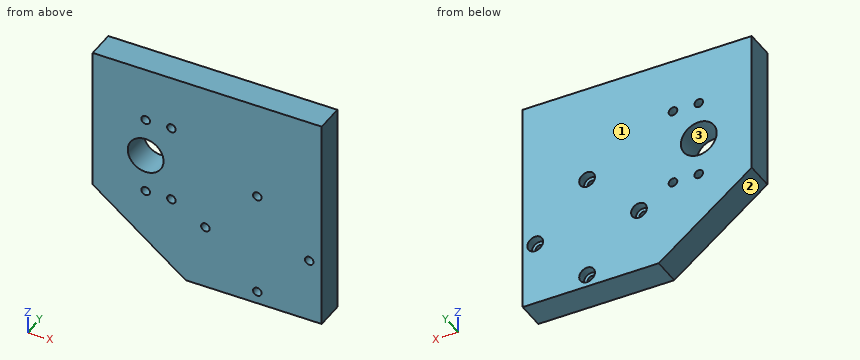
from build123d import *

# Parameters (mm, degrees)
F0_R     = 18
F0_R_2   = 3
F0_W     = 3
F0_H     = 17
F0_H_2   = 27
F0_R_3   = 12.5
F1_DEPTH = 20
F2_DEPTH = 25
F3_R     = 3
F4_DEPTH = 25
F5_R     = 5.5
F6_DEPTH = 6


with BuildPart() as f1:
    # F0 (on Front) → F1 (new body)
    with BuildSketch(Plane.XZ):
        Polygon((60, 50), (60, 0), (155, 0), (155, 90), (63, 90), (63, 63), (60, 63), align=None)
        Polygon((1, 63), (60, 63), (60, 90), (60, 107), (1, 107), align=None)
        with Locations((32, 85)):
            Circle(F0_R, mode=Mode.SUBTRACT)
        Polygon((-5, 50), (60, 50), (60, 63), (1, 63), (1, 107), (60, 107), (60, 120), (-5, 120), align=None)
        with Locations((32, 58)):
            Circle(F0_R_2, mode=Mode.SUBTRACT)
        with Locations((50, 58)):
            Circle(F0_R_2, mode=Mode.SUBTRACT)
        with Locations((32, 112)):
            Circle(F0_R_2, mode=Mode.SUBTRACT)
        with Locations((50, 112)):
            Circle(F0_R_2, mode=Mode.SUBTRACT)
        Polygon((63, 90), (155, 90), (155, 150), (-5, 150), (-5, 120), (60, 120), (60, 107), (63, 107), align=None)
        with Locations((61.5, 98.5)):
            Rectangle(F0_W, F0_H)
        with Locations((61.5, 76.5)):
            Rectangle(F0_W, F0_H_2)
        with Locations((32, 85)):
            Circle(F0_R_3)
        with Locations((32, 85)):
            Circle(F0_R)
        with Locations((32, 85)):
            Circle(F0_R_3, mode=Mode.SUBTRACT)
        Polygon((-5, 50), (60, 0), (60, 50), align=None)
    extrude(amount=F1_DEPTH)

    # F0 (on Front) → F2 (cut)
    with BuildSketch(Plane.XZ):
        with Locations((32, 85)):
            Circle(F0_R_3)
    extrude(amount=F2_DEPTH, mode=Mode.SUBTRACT)

    # F3 (on face) → F4 (cut)
    with BuildSketch(Plane.XZ.offset(20)):
        with Locations((110, 81.25)):
            Circle(F3_R)
        with Locations((146.25, 45)):
            Circle(F3_R)
        with Locations((73.75, 45)):
            Circle(F3_R)
        with Locations((110, 8.75)):
            Circle(F3_R)
    extrude(amount=-F4_DEPTH, mode=Mode.SUBTRACT)

    # F5 (on face) → F6 (cut)
    with BuildSketch(Plane(origin=(0, 0, 0), x_dir=(-1, 0, 0), z_dir=(0, 1, 0))):
        with Locations((-146.25, 45)):
            Circle(F5_R)
        with Locations((-110, 81.25)):
            Circle(F5_R)
        with Locations((-73.75, 45)):
            Circle(F5_R)
        with Locations((-110, 8.75)):
            Circle(F5_R)
    extrude(amount=-F6_DEPTH, mode=Mode.SUBTRACT)


solid = f1.part
Check sheet for the modelled part. Datum: model origin and axes. Units: mm. Face numbers are marked on the shaded views. Round coordinates to 2 decimals unless told otherwise and drop trailing zeros. Order: outer loops, then holes, each group sorted by start corner. A loop starts at its lowest first (then second) coordinate and runs counter-clockwise, first axis right, second up. Notation, with made-up numbers: M 34.5,60.25 L 72.5,60.25 A20 cw 72.5,76.25 Z; hole C 21,35.25 d10. An arc over 180 degrees is marked long. One line per item, written item: value. Start each with the question number.
1. Scan lines: line 1 along Z through (x, y) = (110, -15); line 2 along Z through (x, y) = (146.25, -15.25); line 3 along Z through (x, y) = (50, -8). Record each from-to range of solid material in increasing order.
2. Section check B-B on y = -10.5. Give the number of separate pieces and of enclosed holes in the cut face, and give its area (3 significant figures).
3. Gauge pin test, flat ends, axial feed: P1, Ø15, axis at x = 32, z = 85, coming from the +Y side; P2, Ø9, axis at x = 73.75, z = 45, coming from the +Y side. Record the tip position at first contact, or that the pin passes through.
4. Section check C-C on x = 73.75. Enter the section's corners in (y, z).
5. Section check A-A on z = 45. Enter the section's corners in (x, y), and give its area (3 significant figures).
6. Section check D-D on x = 110. Enter the section's corners in (y, z).
7. Release check for a two-part mould opening along X. For the marked faces 1, 2 and 3 record: released by +X, released by -X, zero draft, split by the parting line, or undercut.
Results found:
1. line 1: 0 to 5.75, 11.75 to 78.25, 84.25 to 150
1. line 2: 0 to 42, 48 to 150
1. line 3: 7.69 to 55, 61 to 109, 115 to 150
2. separate pieces: 1
2. enclosed holes: 9
2. area: 21,700 mm^2
3. P1: through
3. P2: y = -6
4. outline: M -20,0 L 0,0 L 0,39.5 L -6,39.5 L -6,42 L -20,42 Z; M -20,48 L -6,48 L -6,50.5 L 0,50.5 L 0,150 L -20,150 Z
5. outline: M 1.5,-20 L 70.75,-20 L 70.75,-6 L 68.25,-6 L 68.25,0 L 1.5,0 Z; M 76.75,-20 L 143.25,-20 L 143.25,-6 L 140.75,-6 L 140.75,0 L 79.25,0 L 79.25,-6 L 76.75,-6 Z; M 149.25,-20 L 155,-20 L 155,0 L 151.75,0 L 151.75,-6 L 149.25,-6 Z
5. area: 2,770 mm^2
6. outline: M -20,0 L 0,0 L 0,3.25 L -6,3.25 L -6,5.75 L -20,5.75 Z; M -20,11.75 L -6,11.75 L -6,14.25 L 0,14.25 L 0,75.75 L -6,75.75 L -6,78.25 L -20,78.25 Z; M -20,84.25 L -6,84.25 L -6,86.75 L 0,86.75 L 0,150 L -20,150 Z
7. face 1: zero draft
7. face 2: released by -X
7. face 3: undercut
